Can you work these out from the drawing? Everything is in mm from the part's minimum corner. A direction names the side the tool comes from. Round coordinates to 2 decimals unless told otherwise and drop trailing zeros. Loops run counter-clockwise (first coordinate to the right, second up) from the corner with the lowest first, then second, coordinate; pieces in that order, holes last. Notation, with made-up numbers: M 63,44.5 L 108,44.5 A28 ccw 108,71.5 Z; hole C 39,83 d8. An arc over 180 degrees is marked long. Use a Markdown table: item, result.
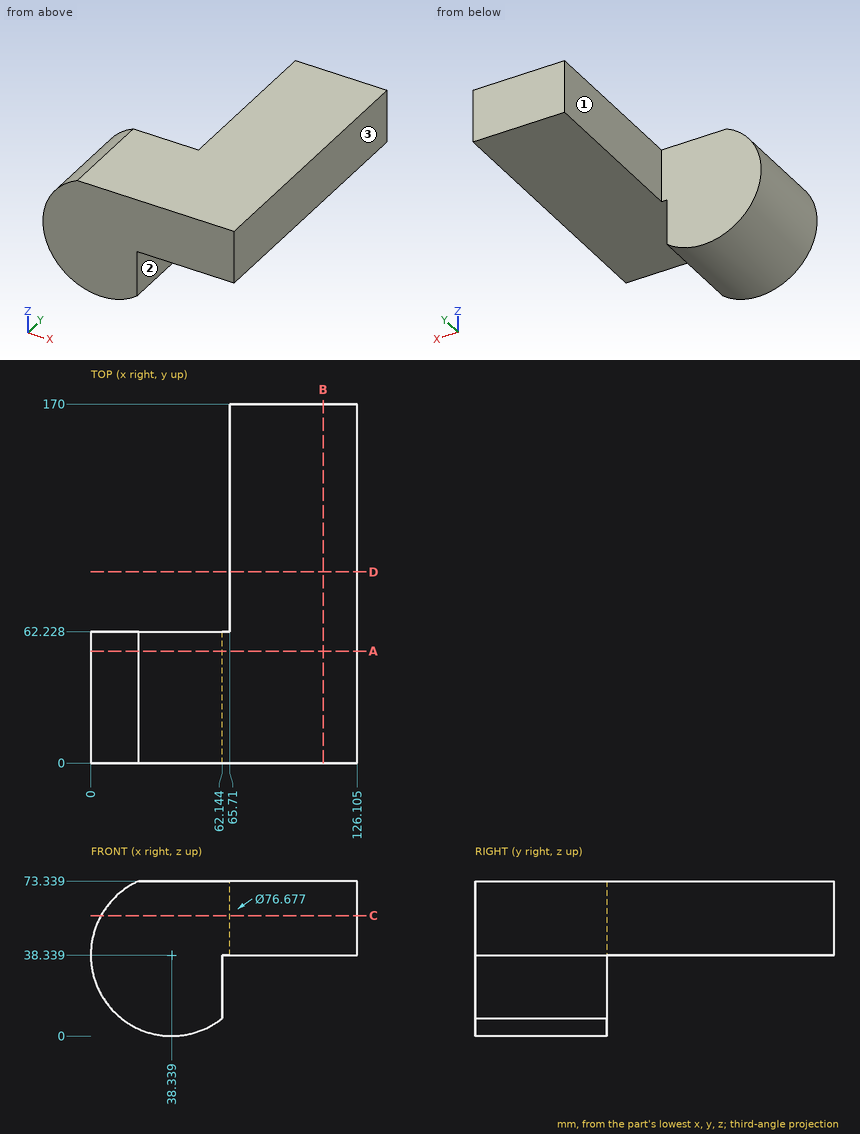
Q1. Will these pins go through, and if not, where does the flat tip stop? P1, Ø6, axis at x = 88.5, y = 97, coming from the -Z side; P2, Ø19.5, axis at x = 19, z = 33, coming from the +Y side; P3, Ø10.5, axis at y = 120.5, z = 48.5, coming from the -X side.
Return value:
| item | result |
|---|---|
| P1 | stops at z = 38.34 |
| P2 | stops at y = 62.23 |
| P3 | stops at x = 65.71 |
Q2. Imagine slicing it at B-B, the plane x = 110. Please give me the cut outline in (y, z), then the cut area to 3 significant figures.
Return value:
| item | result |
|---|---|
| outline | M 0,38.34 L 170,38.34 L 170,73.34 L 0,73.34 Z |
| area | 5,950 mm^2 |
Q3. I need wall thicknesses on line 1 (Z direction, x = 99, y = 53.5); line 2 (Y direction, x = 57.5, z = 5.5); line 3 (X direction, y = 70, z = 61) (1 decimal). Which ranges of each line are inside material? Lowest first, please. Write a range as from..to.
Return value:
| item | result |
|---|---|
| line 1 | z = 38.34..73.34 |
| line 2 | y = 0..62.23 |
| line 3 | x = 65.7..126.1 |
Q4. For the marked faces 1, 2 and 3, which set-ups out of +Z, -Z, +X, -X, +Y, -Y let a thin tool reach every point of the face, with its end or its side?
Return value:
| item | result |
|---|---|
| face 1 | +Z, -Z, -X, +Y |
| face 2 | -Z, +X, +Y, -Y |
| face 3 | +Z, -Z, +X, +Y, -Y |
Q5. Imagine slicing it at C-C, the plane z = 57. Please give me the cut outline in (x, y) (1 decimal).
Return value:
| item | result |
|---|---|
| outline | M 4.8,0 L 126.1,0 L 126.1,170 L 65.7,170 L 65.7,62.2 L 4.8,62.2 Z |
Q6. Imagine slicing it at D-D, the plane y = 90.5. Please give me the cut outline in (x, z) (1 decimal).
Return value:
| item | result |
|---|---|
| outline | M 65.7,38.3 L 126.1,38.3 L 126.1,73.3 L 65.7,73.3 Z |
Q7. Imagine slicing it at A-A, the plane y = 53. Please give me the cut outline in (x, z) (1 decimal), then the cut area to 3 significant figures.
Return value:
| item | result |
|---|---|
| outline | M 22.7,73.3 A38.3 ccw long 62.1,8.3 L 62.1,38.3 L 126.1,38.3 L 126.1,73.3 Z |
| area | 6,200 mm^2 |
